```python
from build123d import *

# Parameters (mm, degrees)
SALIENTE_EXTRUIR1_DEPTH    = 65
VACIADO1_T                 = -5
SALIENTE_EXTRUIR2_DEPTH    = 60
CROQUIS4_W                 = 60.454390592
CROQUIS4_H                 = 25
CORTAR_EXTRUIR1_DEPTH      = 65
CORTAR_EXTRUIR2_DEPTH      = 65
CORTAR_EXTRUIR2_DEPTH_BACK = 75
CROQUIS5_R                 = 7.5
SALIENTE_EXTRUIR3_START    = -7
SALIENTE_EXTRUIR3_DEPTH    = 7
SALIENTE_EXTRUIR5_START    = -7
SALIENTE_EXTRUIR5_DEPTH    = 7
SALIENTE_EXTRUIR7_START    = -7
SALIENTE_EXTRUIR7_DEPTH    = 7
SALIENTE_EXTRUIR8_START    = -7
SALIENTE_EXTRUIR8_DEPTH    = 7
CROQUIS12_R                = 5
CORTAR_EXTRUIR3_DEPTH      = 8


with BuildPart() as part:
    # Croquis2 → Saliente-Extruir1 (new body)
    with BuildSketch(Plane(origin=(0, 0, 0), x_dir=(1, 0, 0), z_dir=(0, 1, 0))):
        with BuildLine():
            ThreePointArc((60, -55), (124.004556318, -18.45744493), (130, 55))
            Line((130, 55), (-130, 55))
            ThreePointArc((-130, 55), (-124.004556318, -18.45744493), (-60, -55))
            Line((-60, -55), (-60, -111.06))
            ThreePointArc((-60, -111.06), (0, -145.004487245), (60, -111.06))
            Line((60, -111.06), (60, -55))
        make_face()
    extrude(amount=SALIENTE_EXTRUIR1_DEPTH)

    # Vaciado1
    vaciado1_openings = [part.faces().sort_by_distance(p)[0] for p in [
        (0, 65, 22.416037692),
    ]]
    offset(amount=VACIADO1_T, openings=vaciado1_openings, kind=Kind.INTERSECTION)

    # Croquis3 → Saliente-Extruir2 (add)
    with BuildSketch(Plane(origin=(0, 5, 0), x_dir=(1, 0, 0), z_dir=(0, 1, 0))):
        with BuildLine():
            ThreePointArc((-60, -49.997006185), (-57.500082648, -50.044139409), (-55, -50.006788897))
            Line((-55, -50.006788897), (-55, -30.006788897))
            Line((-55, -30.006788897), (55, -30.006788897))
            Line((55, -30.006788897), (55, -50.006788897))
            ThreePointArc((55, -50.006788897), (57.500082648, -50.044139409), (60, -49.997006185))
            Line((60, -49.997006185), (60, -25.006788897))
            Line((60, -25.006788897), (-60, -25.006788897))
            Line((-60, -25.006788897), (-60, -49.997006185))
        make_face()
    extrude(amount=SALIENTE_EXTRUIR2_DEPTH)

    # Croquis4 → Cortar-Extruir1 (cut)
    with BuildSketch(Plane.XY.offset(30.006788897)):
        with Locations((1.676963708, 17.5)):
            Rectangle(CROQUIS4_W, CROQUIS4_H)
    extrude(amount=-CORTAR_EXTRUIR1_DEPTH, mode=Mode.SUBTRACT)

    # Croquis5 → Cortar-Extruir2 (cut, two sides: drawn at the far end of the back side and taken through both)
    with BuildSketch(Plane(origin=(130, 0, 0), x_dir=(0, 0, -1), z_dir=(1, 0, 0)).offset(-CORTAR_EXTRUIR2_DEPTH_BACK)):
        with Locations(Location((38.54320604, 13.712018928, 0), (0, 0, 180))):
            Circle(CROQUIS5_R)
    extrude(amount=CORTAR_EXTRUIR2_DEPTH + CORTAR_EXTRUIR2_DEPTH_BACK, mode=Mode.SUBTRACT)

    # Croquis6 → Saliente-Extruir3 (add)
    with BuildSketch(Plane(origin=(0, 65, 0), x_dir=(1, 0, 0), z_dir=(0, 1, 0)).offset(SALIENTE_EXTRUIR3_START)):
        with BuildLine():
            Line((-126.620697254, 50), (-111.620697254, 50))
            Line((-111.620697254, 50), (-111.620697254, 35))
            Line((-111.620697254, 35), (-130.526494323, 35))
            ThreePointArc((-130.526494323, 35), (-128.967419464, 42.602546357), (-126.620697254, 50))
        make_face()
    extrude(amount=SALIENTE_EXTRUIR3_DEPTH)

    # Croquis8 → Saliente-Extruir5 (add)
    with BuildSketch(Plane(origin=(0, 65, 0), x_dir=(1, 0, 0), z_dir=(0, 1, 0)).offset(SALIENTE_EXTRUIR5_START)):
        with BuildLine():
            Line((126.620697254, 50), (111.620697254, 50))
            Line((111.620697254, 50), (111.620697254, 35))
            Line((111.620697254, 35), (130.526494323, 35))
            ThreePointArc((130.526494323, 35), (128.967419464, 42.602546357), (126.620697254, 50))
        make_face()
    extrude(amount=SALIENTE_EXTRUIR5_DEPTH)

    # Croquis10 → Saliente-Extruir7 (add)
    with BuildSketch(Plane(origin=(0, 65, 0), x_dir=(1, 0, 0), z_dir=(0, 1, 0)).offset(SALIENTE_EXTRUIR7_START)):
        with BuildLine():
            Line((-60, -49.997006185), (-60, -34.997006185))
            Line((-60, -34.997006185), (-75, -34.997006185))
            Line((-75, -34.997006185), (-75, -47.909881434))
            ThreePointArc((-75, -47.909881434), (-67.5535332, -49.338182668), (-60, -49.997006185))
        make_face()
    extrude(amount=SALIENTE_EXTRUIR7_DEPTH)

    # Croquis11 → Saliente-Extruir8 (add)
    with BuildSketch(Plane(origin=(0, 65, 0), x_dir=(1, 0, 0), z_dir=(0, 1, 0)).offset(SALIENTE_EXTRUIR8_START)):
        with BuildLine():
            Line((60, -49.997006185), (60, -34.997006185))
            Line((60, -34.997006185), (75, -34.997006185))
            Line((75, -34.997006185), (75, -47.909881434))
            ThreePointArc((75, -47.909881434), (67.5535332, -49.338182668), (60, -49.997006185))
        make_face()
    extrude(amount=SALIENTE_EXTRUIR8_DEPTH)

    # Croquis12 → Cortar-Extruir3 (cut)
    with BuildSketch(Plane(origin=(0, 65, 0), x_dir=(1, 0, 0), z_dir=(0, 1, 0))):
        with Locations(Location((-68, -41.997006185, 0), (0, 0, 270))):
            Circle(CROQUIS12_R)
        with Locations(Location((-118.620697254, 42, 0), (0, 0, 270))):
            Circle(CROQUIS12_R)
        with Locations(Location((118.620697254, 42, 0), (0, 0, 270))):
            Circle(CROQUIS12_R)
        with Locations(Location((68, -41.997006185, 0), (0, 0, 270))):
            Circle(CROQUIS12_R)
    extrude(amount=-CORTAR_EXTRUIR3_DEPTH, mode=Mode.SUBTRACT)


solid = part.part
```
Check sheet for the modelled part. Datum: model origin and axes. Units: mm. A direction names the side the tool comes from. Give positions to 0.01 mm unless a question says otherwise; leave off trailing zeros. Write each loop counter-clockwise with the first axis right and the second up, starting at its lowest first coordinate (ties: lowest second). Pieces come first, ordered by that corner, then holes.
Item 1: Cross-section at D-D (x = 68). Enter the section's corners in (y, z), and give its area (3 significant figures).
Item 2: Cross-section at A-A (y = 24.5). Enter the section's corners in (x, z).
Item 3: Access from +Z, -Z, +X, -X, +Y, -Y to the whole of each face (thin tool, end or side, straight path). Record for faces 1 (the face through (60, 32, 83)), 2 (the face through (60, 35, 38)), 3 (the face through (2, 32, -55)), 4 (the face through (-60, 32, 83)), 5 (the face through (111.621, 61, -43)).
Item 4: Gauge pin test, flat ends, axial feed: pin 1 (16.5 mm diameter, centred on x = -64, z = 46, fed in from -Y); pin 2 (7.5 mm diameter, centred on x = -119.5, y = 63, fed in from +Z); pin 3 (4 mm diameter, centred on y = 23, z = 28, fed in from -X); pin 4 (1 mm diameter, centred on y = 51, z = 83, fed in from -X). Record the tip position at first contact, or that the pin passes through.
Item 5: Cross-section at B-B (y = 41.5). Enter the section's corners in (x, z).
Item 6: Cross-section at C-C (z = 59). Enter the section's corners in (x, y), and give its area (3 significant figures).
Item 7: Scan lines: L1, parallel to Z at x = 41, y = 35; L2, parallel to Z at x = -44, y = 36; L3, parallel to X at y = 10.5, z = 73.5. Record each from-to range of solid material in increasing order.
Item 8: Draft check along Y on faces 6 (the face through (-55, 35, 70)), 7 (the face through (-123, 58, -39)). Enter one of: released by +Y, released by -Y, zero draft, split by the parting line, or undercut.
Report:
1. outline: (0, -55) - (65, -55) - (65, -50) - (5, -50) - (5, 49.27) - (58, 49.27) - (58, 47) - (65, 47) - (65, 54.32) - (0, 54.32) - close; (58, 35) - (65, 35) - (65, 37) - (58, 37) - close
1. area: 1,180 mm2
2. outline: (-130, -55) - (130, -55) arc R79 ccw to (60, 55) - (60, 111.06) arc R70 ccw to (-60, 111.06) - (-60, 55) arc R79 ccw to start; hole (-126.62, -50) - (126.62, -50) arc R74 ccw to (60, 50) - (60, 25.01) - (31.9, 25.01) - (31.9, 30.01) - (55, 30.01) - (55, 109.65) arc R65 ccw to (-55, 109.65) - (-55, 30.01) - (-28.55, 30.01) - (-28.55, 25.01) - (-60, 25.01) - (-60, 50) arc R74 ccw to start
3. face 1: +Z, +X, +Y, -Y
3. face 2: none
3. face 3: -Z, +X, -X, +Y, -Y
3. face 4: +Z, -X, +Y, -Y
3. face 5: +Y
4. pin 1: stops at y = 0
4. pin 2: stops at z = 29.25
4. pin 3: stops at x = -118.56
4. pin 4: stops at x = -60
5. outline: (-130, -55) - (130, -55) arc R79 ccw to (60, 55) - (60, 111.06) arc R70 ccw to (-60, 111.06) - (-60, 55) arc R79 ccw to start; hole (-126.62, -50) - (126.62, -50) arc R74 ccw to (60, 50) - (60, 25.01) - (-60, 25.01) - (-60, 50) arc R74 ccw to start; hole (-55, 30.01) - (55, 30.01) - (55, 109.65) arc R65 ccw to (-55, 109.65) - close
6. outline: (-60, 0) - (60, 0) - (60, 65) - (55, 65) - (55, 5) - (-55, 5) - (-55, 65) - (-60, 65) - close
6. area: 1,200 mm2
7. L1: z = -55 to -50, 25.01 to 30.01, 125.44 to 131.74
7. L2: z = -55 to -50, 25.01 to 30.01, 122.85 to 129.45
7. L3: x = -60 to -55, 55 to 60
8. face 6: zero draft
8. face 7: undercut
